```python
from build123d import *

# Parameters (mm, degrees)
SKETCH1_W           = 241.3
SKETCH1_H           = 76.2
BOSS_EXTRUDE1_DEPTH = 60.325
SKETCH3_W           = 65.0748
SKETCH3_H           = 52.3748
CUT_EXTRUDE4_DEPTH  = 261.136955516
SKETCH6_W           = 95.25
SKETCH6_H           = 52.3748
CUT_EXTRUDE5_DEPTH  = 261.136955516
SKETCH7_W           = 65.0748
SKETCH7_H           = 52.3748
CUT_EXTRUDE6_DEPTH  = 261.136955516
SKETCH8_R           = 6.35
CUT_EXTRUDE7_DEPTH  = 261.136955516
SKETCH9_R           = 9.525
CUT_EXTRUDE8_DEPTH  = 261.136955516
FILLET1_R           = 15.875
FILLET2_R           = 7.9502
FILLET3_R           = 7.9502
FILLET4_R           = 15.875
FILLET5_R           = 15.875
FILLET6_R           = 15.875
FILLET7_R           = 7.9502
FILLET8_R           = 7.9502


with BuildPart() as part:
    # Sketch1 → Boss-Extrude1 (new body)
    with BuildSketch(Plane(origin=(0, 0, 0), x_dir=(1, 0, 0), z_dir=(0, 1, 0))):
        with Locations((120.65, 38.1)):
            Rectangle(SKETCH1_W, SKETCH1_H)
    extrude(amount=BOSS_EXTRUDE1_DEPTH)

    # Sketch3 → Cut-Extrude4 (cut, through all)
    with BuildSketch(Plane.XY):
        with Locations((208.7626, 26.1874)):
            Rectangle(SKETCH3_W, SKETCH3_H)
    extrude(amount=-CUT_EXTRUDE4_DEPTH, mode=Mode.SUBTRACT)

    # Sketch6 → Cut-Extrude5 (cut, through all)
    with BuildSketch(Plane.XY):
        with Locations((120.65, 34.1376)):
            Rectangle(SKETCH6_W, SKETCH6_H)
    extrude(amount=-CUT_EXTRUDE5_DEPTH, mode=Mode.SUBTRACT)

    # Sketch7 → Cut-Extrude6 (cut, through all)
    with BuildSketch(Plane.XY):
        with Locations((32.5374, 26.1874)):
            Rectangle(SKETCH7_W, SKETCH7_H)
    extrude(amount=-CUT_EXTRUDE6_DEPTH, mode=Mode.SUBTRACT)

    # Sketch8 → Cut-Extrude7 (cut, through all)
    with BuildSketch(Plane(origin=(0, 60.325, 0), x_dir=(1, 0, 0), z_dir=(0, 1, 0))):
        with Locations(Location((30.1752, 38.1, 0), (0, 0, 270))):
            Circle(SKETCH8_R)
        with Locations(Location((211.1248, 38.1, 0), (0, 0, 270))):
            Circle(SKETCH8_R)
    extrude(amount=-CUT_EXTRUDE7_DEPTH, mode=Mode.SUBTRACT)

    # Sketch9 → Cut-Extrude8 (cut, through all)
    with BuildSketch(Plane(origin=(0, 60.325, 0), x_dir=(1, 0, 0), z_dir=(0, 1, 0))):
        with Locations(Location((120.65, 38.1, 0), (0, 0, 270))):
            Circle(SKETCH9_R)
    extrude(amount=-CUT_EXTRUDE8_DEPTH, mode=Mode.SUBTRACT)

    # Fillet1
    fillet1_edges = [part.edges().sort_by_distance(p)[0] for p in [
        (73.025, 60.325, -38.1),
    ]]
    fillet(fillet1_edges, radius=FILLET1_R)

    # Fillet2
    fillet2_edges = [part.edges().sort_by_distance(p)[0] for p in [
        (73.025, 7.9502, -38.1),
    ]]
    fillet(fillet2_edges, radius=FILLET2_R)

    # Fillet3
    fillet3_edges = [part.edges().sort_by_distance(p)[0] for p in [
        (168.275, 7.9502, -38.1),
    ]]
    fillet(fillet3_edges, radius=FILLET3_R)

    # Fillet4
    fillet4_edges = [part.edges().sort_by_distance(p)[0] for p in [
        (168.275, 60.325, -38.1),
    ]]
    fillet(fillet4_edges, radius=FILLET4_R)

    # Fillet5
    fillet5_edges = [part.edges().sort_by_distance(p)[0] for p in [
        (176.2252, 0, -38.1),
    ]]
    fillet(fillet5_edges, radius=FILLET5_R)

    # Fillet6
    fillet6_edges = [part.edges().sort_by_distance(p)[0] for p in [
        (65.0748, 0, -38.1),
    ]]
    fillet(fillet6_edges, radius=FILLET6_R)

    # Fillet7
    fillet7_edges = [part.edges().sort_by_distance(p)[0] for p in [
        (65.0748, 52.3748, -38.1),
    ]]
    fillet(fillet7_edges, radius=FILLET7_R)

    # Fillet8
    fillet8_edges = [part.edges().sort_by_distance(p)[0] for p in [
        (176.2252, 52.3748, -38.1),
    ]]
    fillet(fillet8_edges, radius=FILLET8_R)


solid = part.part
```
Design review of the part built by this model. Coordinates are the model's own, in mm. A direction names the side the tool comes from. Coordinates: 2 decimals unless noted, no trailing zeros. Write each loop counter-clockwise with the first axis right and the second up, starting at its lowest first coordinate (ties: lowest second). Pieces come first, ordered by that corner, then holes.
1) Mouldability with a two-part tool opening along Z and no side actions: class faces 1 (the flat face through (111.1, 7.7, 0)), 2 (the cylindrical face through (69.849, 4.527, -38.633)), 3 (the cylindrical face through (123.511, 4.031, -29.015)) as +Z half, -Z half, draft (parallel to the pull), parting line (faces both ways), or undercut.
2) Add section C-C (x = 120.65). Write out the cut boundary in (y, z) (3 decimals), plus the area to 3 significant figures.
3) Add section B-B (z = -38.1). State how many separate pieces and enclosed holes the cut face has, plus the area to 3 significant figures.
4) To check wall thickness, follow L1, parallel to X at y = 15, z = -73; L2, parallel to X at y = 56, z = -38; L3, parallel to X at y = 58.5, z = -38.1. State the ranges of each line that lie inside material, in increasing order.
5) Add section A-A (y = 30). Write out the cut boundary in (x, z) (3 decimals).
6) Insertion check: pin 1 (4 mm diameter, centred on y = 14.5, z = -60.5, fed in from +X); pin 2 (10 mm diameter, centred on x = 30.18, z = -38.1, fed in from -Y); pin 3 (8.5 mm diameter, centred on y = 36.5, z = -53.5, fed in from -X). Each pin has a flat end and moves straight along its axis. Give the tip position at first contact, or say it passes through.
7) Machinability: for faces 4 (the flat face through (219, 52.375, -38)), 5 (the cylindrical face through (75.292, 10.341, -38.633)), 6 (the flat face through (65.075, 30, -38)), which of the approach directions +Z, -Z, +X, -X, +Y, -Y give a long, thin tool a straight path to every point of the face, cutting with its end or side? Answer none if there is none.
8) Add section D-D (z = -23). Write out the cut boundary in (x, y) (3 decimals).
Check result:
1. face 1: +Z half
1. face 2: draft
1. face 3: undercut
2. outline: (0, -76.2) - (7.95, -76.2) - (7.95, -47.625) - (0, -47.625) - close; (0, -28.575) - (7.95, -28.575) - (7.95, 0) - (0, 0) - close
2. area: 454 mm2
3. separate pieces: 4
3. enclosed holes: 0
3. area: 2,240 mm2
4. L1: x = 65.1 to 73.08, 168.22 to 176.2
4. L2: x = 0 to 23.83, 36.52 to 68.04, 173.26 to 204.78, 217.47 to 241.3
4. L3: x = 0 to 23.83, 36.53 to 64.54, 176.76 to 204.77, 217.47 to 241.3
5. outline: (65.075, -76.2) - (73.025, -76.2) - (73.025, 0) - (65.075, 0) - close; (168.275, -76.2) - (176.225, -76.2) - (176.225, 0) - (168.275, 0) - close
6. pin 1: stops at x = 176.23
6. pin 2: passes through
6. pin 3: stops at x = 65.07
7. face 4: +Z, -Z, +X, -Y
7. face 5: +Z, -Z, +Y
7. face 6: +Z, -Z, -X, -Y
8. outline: (0, 52.375) - (57.125, 52.375) arc R7.95 cw to (65.075, 44.425) - (65.075, 15.875) arc R15.875 ccw to (80.95, 0) - (160.35, 0) arc R15.875 ccw to (176.225, 15.875) - (176.225, 44.425) arc R7.95 cw to (184.175, 52.375) - (241.3, 52.375) - (241.3, 60.325) - (184.15, 60.325) arc R15.875 ccw to (168.275, 44.45) - (168.275, 15.9) arc R7.95 cw to (160.325, 7.95) - (80.975, 7.95) arc R7.95 cw to (73.025, 15.9) - (73.025, 44.45) arc R15.875 ccw to (57.15, 60.325) - (0, 60.325) - close
